The listing builds one solid part. Answer for the finished solid, in the listing's coordinates (mm). Face numbers are marked on the shaded views. A direction names the side the tool comes from. Coordinates: 2 decimals unless noted, no trailing zeros. Write each loop counter-clockwise with the first axis right and the second up, starting at its lowest first coordinate (ties: lowest second). Pieces come first, ordered by that corner, then holes. Notation, with made-up numbers: M 38,-34 L 59,-34 A28 cw 59,5 Z; hole C 40,32 d1. An arc over 180 degrees is marked long. Put each result on its own line as item: value. Start each with the question number.
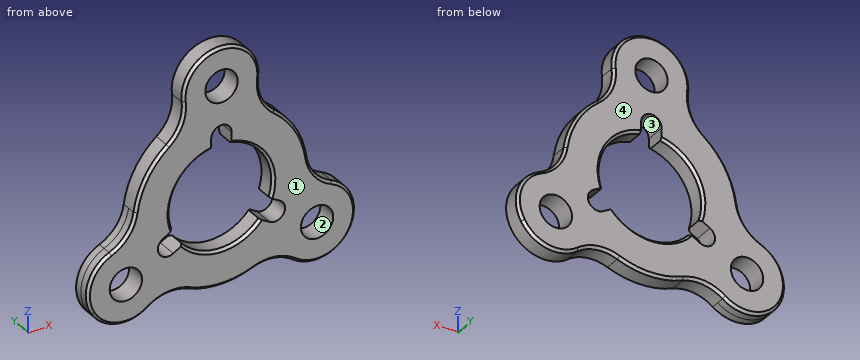
```python
from build123d import *

# Parameters (mm, degrees)
F0_R          = 10
F1_DEPTH      = 2
F1_DEPTH_BACK = 2
F3_D          = 6.3
F4_SIZE       = 0.5
F6_DEPTH      = 4.001


with BuildPart() as f1:
    # F0 (on Front) → F1 (new body, two sides)
    with BuildSketch(Plane.XZ) as f1_sk:
        with BuildLine():
            ThreePointArc((10.4685027699, 13.3944186047), (8.0122088596, 16.6160342353), (7.4491243619, 20.6279069767))
            ThreePointArc((7.4491243619, 20.6279069767), (5.6031552573, 26.4854439284), (0, 29))
            ThreePointArc((0, 29), (-5.6031552573, 26.4854439284), (-7.4491243619, 20.6279069767))
            ThreePointArc((-7.4491243619, 20.6279069767), (-8.0122088596, 16.6160342353), (-10.4685027699, 13.3944186047))
            ThreePointArc((-10.4685027699, 13.3944186047), (-14.7224318643, 8.5), (-16.8341581655, 2.368780036))
            ThreePointArc((-16.8341581655, 2.368780036), (-18.3960121877, -1.3692407048), (-21.5888536497, -3.862822555))
            ThreePointArc((-21.5888536497, -3.862822555), (-25.7386449011, -8.39024717), (-25.1147367097, -14.5))
            ThreePointArc((-25.1147367097, -14.5), (-20.1354896438, -18.0951967583), (-14.1397292878, -16.7650844217))
            ThreePointArc((-14.1397292878, -16.7650844217), (-10.3838033281, -15.2467935304), (-6.3656553956, -15.7631986406))
            ThreePointArc((-6.3656553956, -15.7631986406), (0, -17), (6.3656553956, -15.7631986406))
            ThreePointArc((6.3656553956, -15.7631986406), (10.3838033281, -15.2467935304), (14.1397292878, -16.7650844217))
            ThreePointArc((14.1397292878, -16.7650844217), (20.1354896438, -18.0951967583), (25.1147367097, -14.5))
            ThreePointArc((25.1147367097, -14.5), (25.7386449011, -8.39024717), (21.5888536497, -3.862822555))
            ThreePointArc((21.5888536497, -3.862822555), (18.3960121877, -1.3692407048), (16.8341581655, 2.368780036))
            ThreePointArc((16.8341581655, 2.368780036), (14.7224318643, 8.5), (10.4685027699, 13.3944186047))
        make_face()
        Circle(F0_R, mode=Mode.SUBTRACT)
    extrude(amount=F1_DEPTH)
    extrude(f1_sk.sketch, amount=-F1_DEPTH_BACK)

    # F3 (through all)
    with Locations(Plane.XZ.offset(2)):
        with Locations((0, 21.5), (-18.6195461814, -10.75), (18.6195461814, -10.75)):
            Hole(F3_D / 2)

    # F4
    f4_edges = [f1.edges().sort_by_distance(p)[0] for p in [
        (-10, -2, 0),
        (-10, 2, 0),
        (0, -2, 29),
        (0, 2, 29),
    ]]
    chamfer(f4_edges, length=F4_SIZE)

    # F5 (on face) → F6 (cut, through all)
    with BuildSketch(Plane.XZ.offset(2)):
        with BuildLine():
            ThreePointArc((-2, 9.7979589711), (0, 10), (2, 9.7979589711))
            Line((2, 9.7979589711), (2, 12))
            ThreePointArc((2, 12), (0, 14), (-2, 12))
            Line((-2, 12), (-2, 9.7979589711))
        make_face()
        with BuildLine():
            Line((-9.4852813742, -3.166928678), (-11.3923048454, -4.2679491924))
            ThreePointArc((-11.3923048454, -4.2679491924), (-12.124355653, -7), (-9.3923048454, -7.7320508076))
            Line((-9.3923048454, -7.7320508076), (-7.4852813742, -6.6310302931))
            ThreePointArc((-7.4852813742, -6.6310302931), (-8.6602540378, -5), (-9.4852813742, -3.166928678))
        make_face()
        with BuildLine():
            Line((7.4852813742, -6.6310302931), (9.3923048454, -7.7320508076))
            ThreePointArc((9.3923048454, -7.7320508076), (12.124355653, -7), (11.3923048454, -4.2679491924))
            Line((11.3923048454, -4.2679491924), (9.4852813742, -3.166928678))
            ThreePointArc((9.4852813742, -3.166928678), (8.6602540378, -5), (7.4852813742, -6.6310302931))
        make_face()
    extrude(amount=-F6_DEPTH, mode=Mode.SUBTRACT)


solid = f1.part
```
1) A cutting plane is placed at A-A on x = 0. Write down the section's boundary in (y, z).
2) For the marked faces 3 and 4, determine the directions among +Z, -Z, +X, -X, +Y, -Y from which every point of the face is accessible in a straight line to the end or side of a thin tool.
3) Straight lines are drawn through the part: probe 1 along Z at (x, y) = (0, 0.8); probe 2 along Z at (x, y) = (18.5, -1.2); probe 3 along Z at (x, y) = (0.5, 0.5). For each, find the intervals that lie inside material, in ascending order.
4) Determine the mould class of the marked faces 1 and 2 for opening direction X: +X half, -X half, draft (parallel to the pull), parting line (faces both ways), or undercut.
5) Given pin 1 Ø5.5 at (x, z) = (18.62, -10.75) entering from -Y; pin 2 Ø1 at (x, y) = (-11, 1) entering from +Z; pin 3 Ø1.1 at (y, z) = (-1, 11) entering from -X, each flat-ended and moving along its own axis, determine where each tip first touches the part or whether it passes through.
6) A cutting plane is placed at B-B on y = -0.9. Write down the section's boundary in (x, z), then the cut area to 3 significant figures.
Answers follow:
1. outline: M -2,-16.5 L -1.5,-17 L 1.5,-17 L 2,-16.5 L 2,-10.5 L 1.5,-10 L -1.5,-10 L -2,-10.5 Z; M -2,14 L 2,14 L 2,18.35 L -2,18.35 Z; M -2,24.65 L 2,24.65 L 2,28.5 L 1.5,29 L -1.5,29 L -2,28.5 Z
2. face 3: +Y, -Y
2. face 4: +Z, -Z, +X, -X, +Y
3. probe 1: z = -17 to -10, 14 to 18.35, 24.65 to 29
3. probe 2: z = -18.25 to -13.9, -7.6 to -1.5
3. probe 3: z = -16.99 to -9.99, 13.94 to 18.39, 24.61 to 28.98
4. face 1: draft
4. face 2: undercut
5. pin 1: passes through
5. pin 2: stops at z = 13.37
5. pin 3: stops at x = -13.41
6. outline: M -21.59,-3.86 A7.5 ccw long -14.14,-16.77 A8 cw -6.37,-15.76 A17 ccw 6.37,-15.76 A8 cw 14.14,-16.77 A7.5 ccw long 21.59,-3.86 A8 cw 16.83,2.37 A17 ccw 10.47,13.39 A8 cw 7.45,20.63 A7.5 ccw long -7.45,20.63 A8 cw -10.47,13.39 A17 ccw -16.83,2.37 A8 cw Z; hole C -18.62,-10.75 d6.3; hole M -11.39,-4.27 A2 ccw -9.39,-7.73 L -7.49,-6.63 A10 ccw 7.49,-6.63 L 9.39,-7.73 A2 ccw 11.39,-4.27 L 9.49,-3.17 A10 ccw 2,9.8 L 2,12 A2 ccw -2,12 L -2,9.8 A10 ccw -9.49,-3.17 Z; hole C 0,21.5 d6.3; hole C 18.62,-10.75 d6.3
6. area: 963 mm²
